```python
from build123d import *

# Parameters (mm, degrees)
F0_W     = 50
F0_H     = 40
F2_DEPTH = 20
F1_W     = 20
F1_H     = 10
F3_DEPTH = 20
F4_DEPTH = 20


with BuildPart() as f2:
    # F0 (on Front) → F2 (new body)
    with BuildSketch(Plane.XZ):
        with Locations((21.031922, 2.578686)):
            Rectangle(F0_W, F0_H)
    extrude(amount=F2_DEPTH)

    # F1 (on Front) → F3 (join)
    with BuildSketch(Plane.XZ):
        with Locations((46.17581, 7.295414)):
            Rectangle(F1_W, F1_H)
    extrude(amount=F3_DEPTH)

    # F1 (on Front) → F4 (join)
    with BuildSketch(Plane.XZ):
        Polygon((36.17581, -7.704586), (-3.82419, -7.704586), (-3.82419, -17.704586), (56.17581, -17.704586), (56.17581, -7.704586), align=None)
    extrude(amount=F4_DEPTH)


solid = f2.part
```
The listing builds one solid part. Answer for the finished solid, in the listing's coordinates (mm). A direction names the side the tool comes from. Give positions to 0.01 mm unless a question says otherwise; leave off trailing zeros. Loops run counter-clockwise (first coordinate to the right, second up) from the corner with the lowest first, then second, coordinate; pieces in that order, holes last. Notation, with made-up numbers: M 3,7 L 59,7 A23 cw 59,46 Z; hole C 19.25,9.25 d8. An arc over 180 degrees is marked long. One line per item, written item: value.
1. Find the intervals of material crossed by probe 1 along Z at (x, y) = (50, -7); probe 2 along X at (y, z) = (-5.5, -1.5), in increasing order.
Found:
probe 1: -17.7 to -7.7, 2.3 to 12.3
probe 2: -3.97 to 46.03
2. Each of these flat-tipped pins is pushed along its axis until it touches: P1, Ø2, axis at y = -7.5, z = 16.5, coming from the +X side; P2, Ø5, axis at x = 52, y = -11, coming from the +Z side; P3, Ø8, axis at x = 22, z = 8, coming from the +Y side. Where does it stop, or does it pass through?
Found:
P1: x = 46.03
P2: z = 12.3
P3: y = 0
3. Section A-A on x = 51 is taken. Determine the outline of the cut face in (y, z), plus the area to 3 significant figures.
Found:
outline: M -20,-17.7 L 0,-17.7 L 0,-7.7 L -20,-7.7 Z; M -20,2.3 L 0,2.3 L 0,12.3 L -20,12.3 Z
area: 400 mm^2
4. Section C-C on z = 17 is taken. Determine the outline of the cut face in (x, y).
Found:
outline: M -3.97,-20 L 46.03,-20 L 46.03,0 L -3.97,0 Z
5. For a pull along Z with two mould halves and no side action, classify faces 4 (the face through (51, -10, 2.295)), 5 (the face through (26, -20, 3)), 6 (the face through (21, -10, 22.579)) as pulls with the +Z half, pulls with the -Z half, needs draft (parallel to the pull), parting line crosses it, or undercut.
Found:
face 4: undercut
face 5: needs draft
face 6: pulls with the +Z half
6. Section B-B on y = -1.75 is taken. Determine the outline of the cut face in (x, z).
Found:
outline: M -3.97,-17.42 L -3.82,-17.42 L -3.82,-17.7 L 56.18,-17.7 L 56.18,-7.7 L 46.03,-7.7 L 46.03,2.3 L 56.18,2.3 L 56.18,12.3 L 46.03,12.3 L 46.03,22.58 L -3.97,22.58 Z
7. For faces 1 (the face through (46.032, -10, -3)), 2 (the face through (56.176, -10, 7)), 3 (the face through (51, -10, 12.295)), determine the directions among +Z, -Z, +X, -X, +Y, -Y from which every point of the face is accessible in a straight line to the end or side of a thin tool.
Found:
face 1: +X, +Y, -Y
face 2: +Z, -Z, +X, +Y, -Y
face 3: +Z, +X, +Y, -Y
